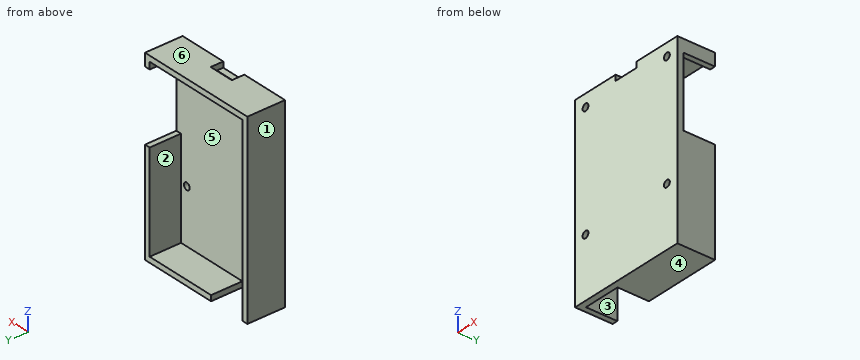
Autodesk Inventor part; units mm, degrees
ref_plane "Work Plane3" through (-25, 0, 42.5) normal (0, -1, 0) x (1, 0, 0)
ref_plane "YZ Plane" through (0, 0, 0) normal (1, 0, 0) x (0, 1, 0)
ref_plane "XZ Plane" through (0, 0, 0) normal (0, 1, 0) x (-1, 0, 0)
ref_plane "Work Plane3" through (-25, 0, 42.5) normal (0, -1, 0) x (1, 0, 0)
sketch "Sketch1" plane through (-25, 0, 42.5) normal (0, -1, 0) x (1, 0, 0)
  line L0 (28.4781, -19.558) -> (28.4781, -33.5534)
  arc A0 (53, -3) -> (50, 0) centre (50, -3) ccw
  line L1 (0, 0) -> (50, 0)
  arc A1 (0, 0) -> (-3, -3) centre (0, -3) ccw
  line L2 (-3, -82) -> (-3, -3)
  arc A2 (-3, -82) -> (0, -85) centre (0, -82) ccw
  line L3 (50, -85) -> (0, -85)
  arc A3 (50, -85) -> (53, -82) centre (50, -82) ccw
  line L4 (53, -3) -> (53, -82)
  circle A4 centre (49.5, -61.5) radius 1.75
  circle A5 centre (0.5, -61.5) radius 1.75
  circle A6 centre (0.5, -3.5) radius 1.75
  circle A7 centre (49.5, -3.5) radius 1.75
  line L5 (-3, 0) -> (53, 0)
  line L6 (53, 0) -> (53, -88.9)
  line L7 (53, -88.9) -> (-3, -88.9)
  line L8 (-3, -88.9) -> (-3, 0)
  point P0 (25, -42.5)
  dimension "d0" = 88.9
extrude "Extrusion1" add sketch "Sketch1" along normal blind 3.175
sketch "Sketch2" plane through (-25, -3.175, 42.5) normal (0, -1, 0) x (1, 0, 0)
  circle A0 centre (49.5, -3.5) radius 1.75
  circle A1 centre (0.5, -3.5) radius 1.75
  circle A2 centre (0.5, -61.5) radius 1.75
  circle A3 centre (49.5, -61.5) radius 1.75
  line L0 (53, 0) -> (-3, 0)
  line L1 (-3, 0) -> (-3, -88.9)
  line L2 (-3, -88.9) -> (53, -88.9)
  line L3 (53, -88.9) -> (53, 0)
  line L4 (-3, -88.9) -> (53, -88.9)
  line L5 (55.8, 2.8) -> (55.8, -91.7)
  line L6 (-5.8, -91.7) -> (-5.8, 2.8)
  line L7 (53, 0) -> (55.8, 2.8)
  line L8 (53, 0) -> (58.3967, 0) construction
  line L9 (55.8, 2.8) -> (-5.8, 2.8)
  line L10 (53, -88.9) -> (61.5609, -88.9) construction
  line L11 (55.8, -91.7) -> (-5.8, -91.7)
  point P0 (25, -42.5)
  dimension "d3" = 45
extrude "Extrusion2" add sketch "Sketch2" against normal blind 19.05 contours L5 L11 L6 L9
sketch "Sketch3" plane through (-25, 15.875, 42.5) normal (0, 1, 0) x (1, 0, 0)
  line L0 (-3, 0) -> (-3, 88.9)
  line L1 (-3, 88.9) -> (53, 88.9)
  line L2 (53, 88.9) -> (53, 0)
  line L3 (53, 0) -> (-3, 0)
  line L4 (-5.8, -2.8) -> (55.8, -2.8)
  line L5 (55.8, -2.8) -> (55.8, 91.7)
  line L6 (55.8, 91.7) -> (-5.8, 91.7)
  line L7 (-5.8, 91.7) -> (-5.8, -2.8)
  line L8 (53, 3.55) -> (55.8, 3.55)
  line L9 (55.8, 3.55) -> (55.8, 39.11)
  line L10 (55.8, 39.11) -> (53, 39.11)
  line L11 (53, 39.11) -> (53, 3.55)
  point P0 (25, 42.5)
  dimension "d7" = 6.35
  dimension "d8" = 35.56
extrude "Extrusion3" cut sketch "Sketch3" against normal blind 15.875 contours L2 L10 L5 L8
sketch "Sketch4" plane through (-25, -3.175, 42.5) normal (0, -1, 0) x (1, 0, 0)
  line L0 (55.8, 2.8) -> (-5.8, 2.8)
  line L1 (18.65, -0.0575) -> (31.35, -0.0575)
  line L2 (31.35, -0.0575) -> (31.35, 2.8)
  line L3 (31.35, 2.8) -> (18.65, 2.8)
  line L4 (18.65, 2.8) -> (18.65, -0.0575)
  line L5 (25, 21.7) -> (25, -110.6)
  point P0 (25, -42.5)
  dimension "d11" = 12.7
  dimension "d12" = 2.8575
extrude "Extrusion4" cut sketch "Sketch4" against normal blind 6.35
sketch "Sketch5" plane through (-25, 15.875, 42.5) normal (0, 1, 0) x (1, 0, 0)
  line L0 (-3, 88.9) -> (16.05, 88.9)
  line L1 (16.05, 88.9) -> (16.05, 91.7575)
  line L2 (16.05, 91.7575) -> (-3, 91.7575)
  line L3 (-3, 91.7575) -> (-3, 88.9)
  line L4 (55.8, 3.55) -> (53, 3.55)
  line L5 (53, 3.55) -> (53, 0)
  line L6 (53, 0) -> (-3, 0)
  line L7 (-3, 0) -> (-3, 88.9)
  line L8 (-3, 88.9) -> (53, 88.9)
  line L9 (53, 88.9) -> (53, 39.11)
  line L10 (53, 39.11) -> (55.8, 39.11)
  line L11 (55.8, 39.11) -> (55.8, 91.7)
  line L12 (55.8, 91.7) -> (-5.8, 91.7)
  line L13 (-5.8, 91.7) -> (-5.8, -2.8)
  line L14 (-5.8, -2.8) -> (55.8, -2.8)
  line L15 (55.8, -2.8) -> (55.8, 3.55)
  point P0 (25, 42.5)
  dimension "d15" = 19.05
  dimension "d16" = 2.8575
  dimension "d17" = 0
extrude "Extrusion5" cut sketch "Sketch5" against normal blind 15.875 contours L3 L12 L1 L0 | L3 L2 L1 L12
properties part number "Raspi3B+_Case"
Input: part model. Units: mm. Frame: model coordinates. Face numbers are marked on the shaded views. A direction names the side the tool comes from. Give positions to 0.01 mm unless a question says otherwise; leave off trailing zeros. Loops run counter-clockwise (first coordinate to the right, second up) from the corner with the lowest first, then second, coordinate; pieces in that order, holes last. Notation, with made-up numbers: (76.25, 88) -> (125.25, 88) arc R19 ccw to (125.25, 97) -> close; hole circle Ø8 at (-31, -14). An arc over 180 degrees is marked (long way). Answer as a JSON object with one key per item and string values. Group by question number.
Item 1: Cut plane D-D, the plane y = 5.75. Return the cut outline in (x, z).
Item 2: Cut plane A-A, the plane x = 24.5. Return the cut outline in (y, z) (3 decimals), and give its area (3 significant figures).
Item 3: Line query: probe 1 along Z at (x, y) = (24.5, -1.5); probe 2 along X at (y, z) = (10.25, -24.5); probe 3 along Z at (x, y) = (26, 5). Output: solid intervals per line, ascending.
Item 4: Pull-direction query (Z, two-part tool) for the marked faces 4, 5 and 6; classes: released by +Z, released by -Z, zero draft, split by the parting line, or undercut.
Item 5: Pin query (flat end, axial travel): P1, Ø5.5, axis at x = 24.5, z = 39, coming from the +Y side; P2, Ø1, axis at y = 8.5, z = 18, coming from the +X side; P3, Ø1.4, axis at x = -2.5, z = 44, coming from the -Y side (3 decimals); P4, Ø3, axis at x = 24.5, z = -19, coming from the -Y side. Return the tip coordinate at first contact, or that it passes through.
Item 6: Cut plane B-B, the plane z = -19. Return the cut outline in (x, y) (3 decimals).
Item 7: Cut plane C-C, the plane x = 0. Return the cut outline in (y, z) (1 decimal).
Item 8: Reachability of the marked faces 1, 2 and 3 from +Z, -Z, +X, -X, +Y, -Y: full face, straight path, thin tool, end or side. Return the list, or none.
Checks:
{
 "1": {"outline": "(-30.8, -49.2) -> (-28, -49.2) -> (-28, 42.5) -> (28, 42.5) -> (28, 38.95) -> (30.8, 38.95) -> (30.8, 45.3) -> (-30.8, 45.3) -> close; (-8.95, -49.2) -> (30.8, -49.2) -> (30.8, 3.39) -> (28, 3.39) -> (28, -46.4) -> (-8.95, -46.4) -> close"},
 "2": {"outline": "(-3.175, -49.2) -> (15.875, -49.2) -> (15.875, -46.4) -> (0, -46.4) -> (0, -20.75) -> (-3.175, -20.75) -> close; (-3.175, -17.25) -> (0, -17.25) -> (0, 37.25) -> (-3.175, 37.25) -> close; (-3.175, 40.75) -> (0, 40.75) -> (0, 42.5) -> (15.875, 42.5) -> (15.875, 45.3) -> (-3.175, 45.3) -> close", "area": "367 mm²"},
 "3": {"probe 1": "z = -49.2 to -20.75, -17.25 to 37.25, 40.75 to 45.3", "probe 2": "x = -30.8 to -28, 28 to 30.8", "probe 3": "z = -49.2 to -46.4, 42.5 to 45.3"},
 "4": {"face 4": "released by -Z", "face 5": "undercut", "face 6": "released by +Z"},
 "5": {"P1": "stops at y = 0", "P2": "stops at x = -28", "P3": "stops at y = 3.175", "P4": "passes through"},
 "6": {"outline": "(-30.8, -3.175) -> (-26.25, -3.175) -> (-26.25, 0) -> (-28, 0) -> (-28, 15.875) -> (-30.8, 15.875) -> close; (-22.75, -3.175) -> (22.75, -3.175) -> (22.75, 0) -> (-22.75, 0) -> close; (26.25, -3.175) -> (30.8, -3.175) -> (30.8, 15.875) -> (28, 15.875) -> (28, 0) -> (26.25, 0) -> close"},
 "7": {"outline": "(-3.2, -49.2) -> (15.9, -49.2) -> (15.9, -46.4) -> (0, -46.4) -> (0, 42.4) -> (-3.2, 42.4) -> close; (3.2, 42.5) -> (15.9, 42.5) -> (15.9, 45.3) -> (3.2, 45.3) -> close"},
 "8": {"face 1": "+Z, -Z, -X, +Y, -Y", "face 2": "+Y", "face 3": "-Z, +Y"}
}
